Build history of the part. All positions in model axes, mm. A direction names the side the tool comes from. Give positions to 0.01 mm unless a question says otherwise; leave off trailing zeros. Order: outer loops, then holes, each group sorted by start corner. A loop starts at its lowest first (then second) coordinate and runs counter-clockwise, first axis right, second up. Notation, with made-up numbers: (37, 20.5) -> (71, 20.5) arc R9 cw to (71, 36.5) -> close; hole circle Ø7 at (50, 88). An arc over 180 degrees is marked (long way). Use a Markdown table: item, result. Add a question column.
```python
from build123d import *

# Parameters (mm, degrees)
CROQUIS1_W                 = 107
CROQUIS1_H                 = 115.41
CROQUIS1_R                 = 2
SALIENTE_EXTRUIR1_DEPTH    = 6
CROQUIS2_W                 = 115
CROQUIS2_H                 = 123.41
CROQUIS2_W_2               = 107
CROQUIS2_H_2               = 115.41
SALIENTE_EXTRUIR2_DEPTH    = 70
CROQUIS3_R                 = 7.5
CORTAR_EXTRUIR1_DEPTH      = 51
CORTAR_EXTRUIR2_DEPTH      = 166
CORTAR_EXTRUIR2_DEPTH_BACK = 31
CROQUIS4_R                 = 1.75
CROQUIS4_W                 = 21
CROQUIS4_H                 = 16.5
CROQUIS6_W                 = 17
CROQUIS6_H                 = 12
CORTAR_EXTRUIR3_DEPTH      = 3
CORTAR_EXTRUIR4_DEPTH      = 18
CORTAR_EXTRUIR4_DEPTH_BACK = 21
CROQUIS8_W                 = 30
CROQUIS8_H                 = 40
CORTAR_EXTRUIR5_DEPTH      = 1
CROQUIS9_R                 = 5
CROQUIS9_R_2               = 1.999291975
CROQUIS9_R_3               = 2
SALIENTE_EXTRUIR3_DEPTH    = 12
CROQUIS10_R                = 3.5
CORTAR_EXTRUIR6_DEPTH      = 3
CROQUIS11_R                = 3.5
CROQUIS11_R_2              = 1.75
SALIENTE_EXTRUIR4_DEPTH    = 68
CROQUIS12_R                = 5
CROQUIS12_R_2              = 8
SALIENTE_EXTRUIR5_DEPTH    = 6
CROQUIS13_R                = 2.5
CROQUIS13_W                = 18
CROQUIS13_H                = 30
CORTAR_EXTRUIR7_DEPTH      = 10


with BuildPart() as part:
    # Croquis1 → Saliente-Extruir1 (new body)
    with BuildSketch(Plane.XY):
        with Locations((31.5, 35.705)):
            Rectangle(CROQUIS1_W, CROQUIS1_H)
        Circle(CROQUIS1_R, mode=Mode.SUBTRACT)
        with Locations((38, 0)):
            Circle(CROQUIS1_R, mode=Mode.SUBTRACT)
        with Locations((38, 71.41)):
            Circle(CROQUIS1_R, mode=Mode.SUBTRACT)
    extrude(amount=SALIENTE_EXTRUIR1_DEPTH)

    # Croquis2 → Saliente-Extruir2 (add)
    with BuildSketch(Plane.XY):
        with Locations((31.5, 35.705)):
            Rectangle(CROQUIS2_W, CROQUIS2_H)
        with Locations((31.5, 35.705)):
            Rectangle(CROQUIS2_W_2, CROQUIS2_H_2, mode=Mode.SUBTRACT)
    extrude(amount=SALIENTE_EXTRUIR2_DEPTH)

    # Croquis3 → Cortar-Extruir1 (cut)
    with BuildSketch(Plane(origin=(90, 0, 0), x_dir=(0, 0, -1), z_dir=(1, 0, 0))):
        with Locations(Location((-45, 77.41, 0), (0, 0, 180))):
            Circle(CROQUIS3_R)
        with Locations(Location((-45, -6, 0), (0, 0, 180))):
            Circle(CROQUIS3_R)
        with BuildLine():
            Line((-14.5, -1), (-25.5, -1))
            ThreePointArc((-25.5, -1), (-26.914213562, -1.585786438), (-27.5, -3))
            Line((-27.5, -3), (-27.5, -9))
            ThreePointArc((-27.5, -9), (-26.914213562, -10.414213562), (-25.5, -11))
            Line((-25.5, -11), (-14.5, -11))
            ThreePointArc((-14.5, -11), (-13.085786438, -10.414213562), (-12.5, -9))
            Line((-12.5, -9), (-12.5, -3))
            ThreePointArc((-12.5, -3), (-13.085786438, -1.585786438), (-14.5, -1))
        make_face()
        with BuildLine():
            Line((-29, 84.41), (-11, 84.41))
            ThreePointArc((-11, 84.41), (-9.585786438, 83.824213562), (-9, 82.41))
            Line((-9, 82.41), (-9, 72.41))
            ThreePointArc((-9, 72.41), (-9.585786438, 70.995786438), (-11, 70.41))
            Line((-11, 70.41), (-29, 70.41))
            ThreePointArc((-29, 70.41), (-30.414213562, 70.995786438), (-31, 72.41))
            Line((-31, 72.41), (-31, 82.41))
            ThreePointArc((-31, 82.41), (-30.414213562, 83.824213562), (-29, 84.41))
        make_face()
    extrude(amount=-CORTAR_EXTRUIR1_DEPTH, mode=Mode.SUBTRACT)

    # Croquis4 → Cortar-Extruir2 (cut, two sides: drawn at the far end of the back side and taken through both)
    with BuildSketch(Plane(origin=(0, -30, 0), x_dir=(1, 0, 0), z_dir=(0, 1, 0)).offset(-CORTAR_EXTRUIR2_DEPTH_BACK)):
        with Locations(Location((19, -35, 0), (0, 0, 90))):
            Circle(CROQUIS4_R)
        with Locations((31.5, -35)):
            Rectangle(CROQUIS4_W, CROQUIS4_H)
    extrude(amount=CORTAR_EXTRUIR2_DEPTH + CORTAR_EXTRUIR2_DEPTH_BACK, mode=Mode.SUBTRACT)

    # Croquis6 → Cortar-Extruir3 (cut)
    with BuildSketch(Plane(origin=(-26, 0, 0), x_dir=(0, 0, -1), z_dir=(1, 0, 0))):
        with Locations((-35, 35.705)):
            Rectangle(CROQUIS6_W, CROQUIS6_H)
    extrude(amount=CORTAR_EXTRUIR3_DEPTH, mode=Mode.SUBTRACT)

    # Croquis7 → Cortar-Extruir4 (cut, two sides: drawn at the far end of the back side and taken through both)
    with BuildSketch(Plane(origin=(-26, 0, 0), x_dir=(0, 0, -1), z_dir=(1, 0, 0)).offset(-CORTAR_EXTRUIR4_DEPTH_BACK)):
        Polygon((-43.5, 41.705), (-40.5, 41.705), (-39.5, 41.705), (-39.5, 29.705), (-40.5, 29.705), (-43.5, 29.705), align=None)
    extrude(amount=CORTAR_EXTRUIR4_DEPTH + CORTAR_EXTRUIR4_DEPTH_BACK, mode=Mode.SUBTRACT)

    # Croquis8 → Cortar-Extruir5 (cut)
    with BuildSketch(Plane(origin=(-26, 0, 0), x_dir=(0, 0, -1), z_dir=(1, 0, 0))):
        with Locations((-35, 35.705)):
            Rectangle(CROQUIS8_W, CROQUIS8_H)
    extrude(amount=CORTAR_EXTRUIR5_DEPTH, mode=Mode.SUBTRACT)

    # Croquis9 → Saliente-Extruir3 (add)
    # profile 1 of 3: a face of its own
    with BuildSketch(Plane.XY):
        with Locations(Location((38, 0, 0), (0, 0, 180))):
            Circle(CROQUIS9_R)
        with Locations((38, 0)):
            Circle(CROQUIS9_R_2, mode=Mode.SUBTRACT)
    # profile 2 of 3: a face of its own
    with BuildSketch(Plane.XY):
        with Locations(Location((0, 0, 0), (0, 0, 180))):
            Circle(CROQUIS9_R)
        Circle(CROQUIS9_R_3, mode=Mode.SUBTRACT)
    # profile 3 of 3: a face of its own
    with BuildSketch(Plane.XY):
        with Locations(Location((38, 71.41, 0), (0, 0, 180))):
            Circle(CROQUIS9_R)
        with Locations((38, 71.41)):
            Circle(CROQUIS9_R_3, mode=Mode.SUBTRACT)
    extrude(amount=SALIENTE_EXTRUIR3_DEPTH)

    # Croquis10 → Cortar-Extruir6 (cut)
    with BuildSketch(Plane.XY):
        with Locations((38, 71.41)):
            Circle(CROQUIS10_R)
        Circle(CROQUIS10_R)
        with Locations((38, 0)):
            Circle(CROQUIS10_R)
    extrude(amount=CORTAR_EXTRUIR6_DEPTH, mode=Mode.SUBTRACT)

    # Croquis11 → Saliente-Extruir4 (add)
    # profile 1 of 4: a face of its own
    with BuildSketch(Plane.XY):
        with Locations((-19, -19)):
            Circle(CROQUIS11_R)
        with Locations(Location((-19, -19, 0), (0, 0, 180))):
            Circle(CROQUIS11_R_2, mode=Mode.SUBTRACT)
    # profile 2 of 4: a face of its own
    with BuildSketch(Plane.XY):
        with Locations((-19, 90.41)):
            Circle(CROQUIS11_R)
        with Locations(Location((-19, 90.41, 0), (0, 0, 180))):
            Circle(CROQUIS11_R_2, mode=Mode.SUBTRACT)
    # profile 3 of 4: a face of its own
    with BuildSketch(Plane.XY):
        with Locations((82, 90.41)):
            Circle(CROQUIS11_R)
        with Locations(Location((82, 90.41, 0), (0, 0, 180))):
            Circle(CROQUIS11_R_2, mode=Mode.SUBTRACT)
    # profile 4 of 4: a face of its own
    with BuildSketch(Plane.XY):
        with Locations((82, -19)):
            Circle(CROQUIS11_R)
        with Locations(Location((82, -19, 0), (0, 0, 180))):
            Circle(CROQUIS11_R_2, mode=Mode.SUBTRACT)
    extrude(amount=SALIENTE_EXTRUIR4_DEPTH)

    # Croquis12 → Saliente-Extruir5 (add)
    # profile 1 of 2: a face of its own
    with BuildSketch(Plane.XY):
        Polygon((64, 97.41), (-1, 97.41), (-1, 107.41), (-26, 107.41), (-26, 117.41), (6.5, 132.41), (56.5, 132.41), (89, 117.41), (89, 107.41), (64, 107.41), align=None)
        with Locations((56.5, 117.41)):
            Circle(CROQUIS12_R, mode=Mode.SUBTRACT)
        with Locations((6.5, 117.41)):
            Circle(CROQUIS12_R, mode=Mode.SUBTRACT)
        with Locations((31.5, 117.41)):
            Circle(CROQUIS12_R_2, mode=Mode.SUBTRACT)
    # profile 2 of 2: a face of its own
    with BuildSketch(Plane.XY):
        Polygon((-1, -36), (-26, -36), (-26, -46), (6.5, -61), (56.5, -61), (89, -46), (89, -36), (64, -36), (64, -26), (-1, -26), align=None)
        with Locations((56.5, -46)):
            Circle(CROQUIS12_R, mode=Mode.SUBTRACT)
        with Locations((31.5, -46)):
            Circle(CROQUIS12_R_2, mode=Mode.SUBTRACT)
        with Locations((6.5, -46)):
            Circle(CROQUIS12_R, mode=Mode.SUBTRACT)
    extrude(amount=SALIENTE_EXTRUIR5_DEPTH)

    # Croquis13 → Cortar-Extruir7 (cut)
    with BuildSketch(Plane(origin=(90, 0, 0), x_dir=(0, 0, -1), z_dir=(1, 0, 0))):
        with Locations(Location((-30, 13.705, 0), (0, 0, 180))):
            Circle(CROQUIS13_R)
        with Locations(Location((-30, 57.705, 0), (0, 0, 180))):
            Circle(CROQUIS13_R)
        with Locations((-30, 35.705)):
            Rectangle(CROQUIS13_W, CROQUIS13_H)
    extrude(amount=-CORTAR_EXTRUIR7_DEPTH, mode=Mode.SUBTRACT)


solid = part.part
```
(1) Band-saw the part on C-C on y = 103. Give the cut face in (x, z).
(2) Tool access for faces 1 (the face through (77, 107.41, 3)), 2 (the face through (87, 77, 9)), 3 (the face through (38, 74, 12)): list every direction of +Z, -Z, +X, -X, +Y, -Y with a clear straight run to the whole face (end or side of a thin tool).
(3) Band-saw the part on B-B on z = 61.5. State how many separate pieces and enclosed holes the cut face has, plus the area to 3 significant figures.
(4) Band-saw the part on A-A on x = 14.5. Give the cut face in (y, z).
(5) Pin check, flat tips, straight feed: pin 1 Ø4.5 at (y, z) = (13.705, 30) entering from +X; pin 2 Ø9.5 at (x, y) = (31.5, -46) entering from +Z; pin 3 Ø3 at (x, y) = (28.5, 33) entering from +Z; pin 4 Ø3 at (x, y) = (38, 69.5) entering from +Z. Stop position of each tip, or through.
(6) Wall check: probe 1 along X at (y, z) = (-23, 35); probe 2 along Y at (x, z) = (-19, 29.5); probe 3 along Y at (x, z) = (56.5, 1.6). Give the ranges that are in metal, low to high.
(7) Mould opens along X. For faces 4 (the face through (87, -11, 20)), 5 (the face through (79.46, 88, 36.57)) say: released by +X, released by -X, zero draft, split by the parting line, or undercut.
Response:
| question | item | result |
|---|---|---|
| 1 | outline | (-1, 0) -> (64, 0) -> (64, 6) -> (-1, 6) -> close |
| 2 | face 1 | +Z, -Z, +X |
| 2 | face 2 | +X |
| 2 | face 3 | +Z |
| 3 | separate pieces | 1 |
| 3 | enclosed holes | 9 |
| 3 | area | 1,950 mm² |
| 4 | outline | (-61, 0) -> (132.41, 0) -> (132.41, 6) -> (97.41, 6) -> (97.41, 70) -> (93.41, 70) -> (93.41, 6) -> (-22, 6) -> (-22, 70) -> (-26, 70) -> (-26, 6) -> (-61, 6) -> close |
| 5 | pin 1 | stops at x = -22 |
| 5 | pin 2 | passes through |
| 5 | pin 3 | stops at z = 6 |
| 5 | pin 4 | stops at z = 12 |
| 6 | probe 1 | x = -26 to 17.25, 20.75 to 21, 42 to 89 |
| 6 | probe 2 | y = -26 to -20.75, -17.25 to -15.5, 86.91 to 88.66, 92.16 to 97.41 |
| 6 | probe 3 | y = -61 to -51, -41 to 112.41, 122.41 to 132.41 |
| 7 | face 4 | zero draft |
| 7 | face 5 | undercut |
